```python
from build123d import *

# Parameters (mm, degrees)
F0_R     = 7.9375
F1_DEPTH = 41.529
F4_DEPTH = 3.175
F5_W     = 1.8542
F5_H     = 3.048
F7_SIZE  = 0.508


with BuildPart() as f1:
    # F0 (on Front) → F1 (new body)
    with BuildSketch(Plane.XZ):
        Circle(F0_R)
    extrude(amount=F1_DEPTH)

    # F3 (on offset) → F4 (cut)
    with BuildSketch(Plane.XY.offset(9.398)):
        with BuildLine():
            Line((2.413, -20.32), (2.413, 0))
            Line((2.413, 0), (-2.413, 0))
            Line((-2.413, 0), (-2.413, -20.32))
            ThreePointArc((-2.413, -20.32), (0, -22.733), (2.413, -20.32))
        make_face()
    extrude(amount=-F4_DEPTH, mode=Mode.SUBTRACT)

    # F5 (on Right) → F6 (revolve, cut)
    with BuildSketch(Plane.YZ):
        with Locations((-2.5781, 8.500982)):
            Rectangle(F5_W, F5_H)
    revolve(axis=Axis((0, 0, 0), (0, -1, 0)), mode=Mode.SUBTRACT)

    # F7
    f7_edges = [f1.edges().sort_by_distance(p)[0] for p in [
        (-7.9375, -41.529, 0),
        (0, 0, -7.9375),
    ]]
    chamfer(f7_edges, length=F7_SIZE)


solid = f1.part
```
Input: part model. Units: mm. Frame: model coordinates. A direction names the side the tool comes from. Coordinates: 2 decimals unless noted, no trailing zeros. Loops run counter-clockwise (first coordinate to the right, second up) from the corner with the lowest first, then second, coordinate; pieces in that order, holes last. Notation, with made-up numbers: (36, -14.75) - (43, -14.75) arc R25 ccw to (43, 23.25) - close; hole circle Ø6 at (35.25, 14.25). An arc over 180 degrees is marked (long way). Answer in a Markdown table with one row per item.
(1) Pin query (flat end, axial travel): P1, Ø6, axis at x = -3, y = -28, coming from the -Z side; P2, Ø2, axis at x = -4.5, y = -20, coming from the -Z side; P3, Ø5.5, axis at x = -1, y = -9, coming from the +Z side; P4, Ø1.1, axis at y = -7, z = 7, coming from the -X side. Return the tip coordinate at first contact, or that it passes through.
Model answer:
| item | result |
|---|---|
| P1 | stops at z = -7.94 |
| P2 | stops at z = -7.12 |
| P3 | stops at z = 7.56 |
| P4 | stops at x = -4.63 |
(2) Cut plane B-B on y = -31. Output: boundary loops of the cut face in (x, z) (1 decimal).
Model answer:
| item | result |
|---|---|
| outline | circle Ø15.9 at (0, 0) |
(3) Cut plane A-A on x = 0. Output: boundary loops of the cut face in (y, z).
Model answer:
| item | result |
|---|---|
| outline | (-41.53, -7.43) - (-41.02, -7.94) - (-3.51, -7.94) - (-3.51, -6.98) - (-1.65, -6.98) - (-1.65, -7.94) - (-0.51, -7.94) - (0, -7.43) - (0, 6.22) - (-22.73, 6.22) - (-22.73, 7.94) - (-41.02, 7.94) - (-41.53, 7.43) - close |
(4) Set-up query: faces 1 (the face through (-0.31, -1.07, -7.93)), 2 (the face through (-0.053, -22.732, 6.906)), 3 (the face through (-1.21, -1.651, -7.04)). Return all of +Z, -Z, +X, -X, +Y, -Y with unobstructed straight access to the full face (end or side cutting, diameter ignored); none if empty.
Model answer:
| item | result |
|---|---|
| face 1 | +Y, -Y |
| face 2 | +Z, +Y |
| face 3 | none |
(5) Cut plane C-C on y = -19. Output: boundary loops of the cut face in (x, z) (1 decimal), plus the area to 3 significant figures.
Model answer:
| item | result |
|---|---|
| outline | (-2.4, 6.2) - (-2.4, 7.6) arc R7.9 ccw (long way) to (2.4, 7.6) - (2.4, 6.2) - close |
| area | 190 mm² |
(6) Material intervals for L1, parallel to Y at x = -2.75, z = 6.75; L2, parallel to X at y = -6, z = 6.75; L3, parallel to Y at x = 7, z = -3.25, sorted ascending. Write a range as from..to.
Model answer:
| item | result |
|---|---|
| L1 | y = -41.53..-3.51, -1.65..0 |
| L2 | x = -4.18..-2.41, 2.41..4.18 |
| L3 | y = -41.24..-3.51, -1.65..-0.29 |
(7) Mould query, pull axis X, two halves, no side actions, for faces 4 (the face through (0, -11, 6.223)), 5 (the face through (-1.72, -22, -7.75)), 6 (the face through (0, -41.529, 0)). Classes: pulls with the +X half, pulls with the -X half, needs draft (parallel to the pull), parting line crosses it, or undercut.
Model answer:
| item | result |
|---|---|
| face 4 | undercut |
| face 5 | parting line crosses it |
| face 6 | needs draft |
